Design review of the part built by this model. Coordinates are the model's own, in mm. Face numbers are marked on the shaded views. A direction names the side the tool comes from. Coordinates: 2 decimals unless noted, no trailing zeros. Loops run counter-clockwise (first coordinate to the right, second up) from the corner with the lowest first, then second, coordinate; pieces in that order, holes last. Notation, with made-up numbers: (-21, -21) -> (26, -21) arc R21 cw to (26, -11) -> close; hole circle Ø2 at (81.5, 46.25). An arc over 180 degrees is marked (long way). Use CSV: the item, a comma, the result in double quotes.
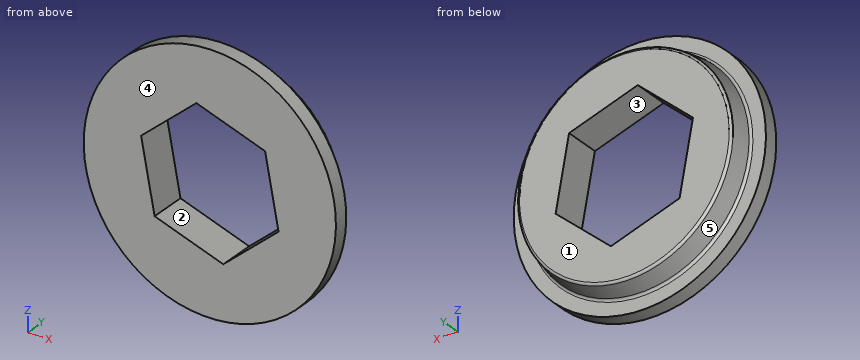
```python
from build123d import *

# Parameters (mm, degrees)
CUT_EXTRUDE1_DEPTH = 19.360177014
FILLET1_R          = 0.254


with BuildPart() as part:
    # Sketch1 → Revolve1 (revolve)
    with BuildSketch(Plane(origin=(0, 0, 0), x_dir=(0, 0, -1), z_dir=(1, 0, 0)), mode=Mode.PRIVATE) as revolve1_sk:
        Polygon((0, 3.81), (10.772916522, 3.81), (11.176, 1.524), (12.7, 1.524), (12.7, 0), (0, 0), align=None)
    revolve(revolve1_sk.sketch.rotate(Axis((0, 8.524875, 0), (0, -1, 0)), 180), axis=Axis((0, 8.524875, 0), (0, -1, 0)))

    # Sketch2 → Cut-Extrude1 (cut, through all)
    with BuildSketch(Plane(origin=(0, 3.81, 0), x_dir=(1, 0, 0), z_dir=(0, 1, 0))):
        Polygon((5.563452778, -4.776120446), (6.917968027, 2.430031215), (1.354515249, 7.206151662), (-5.563452778, 4.776120446), (-6.917968027, -2.430031215), (-1.354515249, -7.206151662), align=None)
    extrude(amount=-CUT_EXTRUDE1_DEPTH, mode=Mode.SUBTRACT)

    # Fillet1
    fillet1_edges = [part.edges().sort_by_distance(p)[0] for p in [
        (0, 1.524, -11.176),
        (0, 3.81, -10.772916522),
    ]]
    fillet(fillet1_edges, radius=FILLET1_R)


solid = part.part
```
Item 1: Add section A-A (y = 2.3). Give the boundary of the cut face in (x, z).
Checked values:
outline,"circle Ø22.08 at (0, 0); hole (-6.92, 2.43) -> (-5.56, -4.78) -> (1.35, -7.21) -> (6.92, -2.43) -> (5.56, 4.78) -> (-1.35, 7.21) -> close"
Item 2: Add section B-B (z = 0). Give the boundary of the cut face in (x, y), then the cut area to 3 significant figures.
Checked values:
outline,"(-12.7, 0) -> (-6.46, 0) -> (-6.46, 3.81) -> (-10.56, 3.81) arc R0.25 ccw to (-10.81, 3.6) -> (-11.14, 1.73) arc R0.25 cw to (-11.39, 1.52) -> (-12.7, 1.52) -> close; (6.46, 0) -> (12.7, 0) -> (12.7, 1.52) -> (11.39, 1.52) arc R0.25 cw to (11.14, 1.73) -> (10.81, 3.6) arc R0.25 ccw to (10.56, 3.81) -> (6.46, 3.81) -> close"
area,"39.7 mm^2"
Item 3: Add section C-C (x = 0). Give the boundary of the cut face in (y, z).
Checked values:
outline,"(0, -12.7) -> (1.52, -12.7) -> (1.52, -11.39) arc R0.25 cw to (1.73, -11.14) -> (3.6, -10.81) arc R0.25 ccw to (3.81, -10.56) -> (3.81, -6.73) -> (0, -6.73) -> close; (0, 6.73) -> (3.81, 6.73) -> (3.81, 10.56) arc R0.25 ccw to (3.6, 10.81) -> (1.73, 11.14) arc R0.25 cw to (1.52, 11.39) -> (1.52, 12.7) -> (0, 12.7) -> close"
Item 4: Clearance check with flat-ended pins moving along their axes: pin 1 (2 mm diameter, centred on y = 3, z = 8, fed in from +X); pin 2 (1.5 mm diameter, centred on x = 4, y = 3.5, fed in from -Z). State where each tip first meets the part, or that it passes through.
Checked values:
pin 1,"x = 8.41"
pin 2,"z = -10.37"
Item 5: To check wall thickness, follow line 1 along X through (y, z) = (3.2, -3.75); line 2 along X through (y, z) = (1.7, 2.5); line 3 along Z through (x, y) = (4.5, 0.55). State the ranges of each line that lie inside material, in increasing order.
Checked values:
line 1,"-10.21 to -5.76, 5.38 to 10.21"
line 2,"-10.86 to -6.84, 5.99 to 10.86"
line 3,"-11.88 to -4.51, 5.15 to 11.88"
Item 6: Machinability: for the marked faces 1 and 2, which of the approach directions +Z, -Z, +X, -X, +Y, -Y give a long, thin tool a straight path to every point of the face, cutting with its end or side? Answer none if there is none.
Checked values:
face 1,"+Z, -Z, +X, -X, +Y"
face 2,"+Y, -Y"
Item 7: Draft analysis for pull direction Z (two halves, no side actions). For the marked faces 3, 4 and 5, state which applies: pulls with the +Z half, pulls with the -Z half, needs draft (parallel to the pull), parting line crosses it, or undercut.
Checked values:
face 3,"undercut"
face 4,"needs draft"
face 5,"parting line crosses it"
